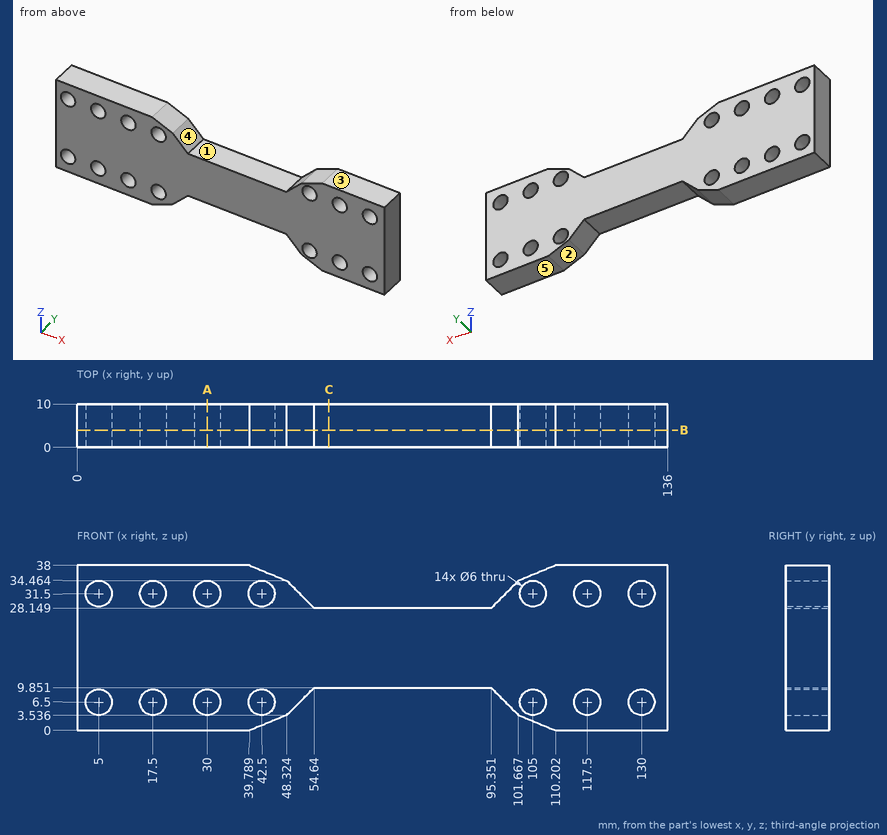
Part print with two shaded views. Sizes in mm from the minimum x, y, z corner. A direction names the side the tool comes from. Coordinates: 2 decimals unless noted, no trailing zeros. Order: outer loops, then holes, each group sorted by start corner. A loop starts at its lowest first (then second) coordinate and runs counter-clockwise, first axis right, second up. Notation, with made-up numbers: (-13.5, 39) - (22.5, 39) arc R16 cw to (22.5, 47) - close; hole circle Ø1 at (59.5, 53). An arc over 180 degrees is marked (long way). Write item = value, one per line. Start each with the question number.
1) Two-plate mould, pull along X, no slides. Class the marked faces 4 and 5: pulls with the +X half, pulls with the -X half, needs draft (parallel to the pull), parting line crosses it, or undercut.
2) Wall check: line 1 along Z through (x, y) = (44, 4) (1 decimal); line 2 along Z through (x, y) = (120, 6.75) (1 decimal); line 3 along Z through (x, y) = (57, 9.25). Give the ranges that are in metal, low to high. Write a range as from..to.
3) Flat gauge pins, fed straight in: pin 1 Ø5 at (x, z) = (30, 31.5) entering from -Y; pin 2 Ø3 at (x, y) = (72.5, 9) entering from -Z; pin 3 Ø5 at (x, y) = (71, 7.5) entering from +Z. Where does each tip first touch, or does it go through?
4) Saw through at B-B on y = 4. Count the separate pieces of the cut face and the enclosed holes in it, then the cut area to 3 significant figures.
5) 3-axis set-ups, long thin cutter, end or side, ignore diameter. For the marked faces 1, 2 and 3: which of +Z, -Z, +X, -X, +Y, -Y reach the whole face in a straight line?
6) Saw through at C-C on x = 58. Write the cut outline in (y, z), then the cut area to 3 significant figures.
7) Saw through at A-A on x = 30. Write the cut outline in (y, z), then the cut area to 3 significant figures.
From the geometry:
q1.face_4 = undercut
q1.face_5 = needs draft
q2.line_1 = 1.7..3.9, 9.1..28.9, 34.1..36.3
q2.line_2 = 0..4.8, 8.2..29.8, 33.2..38
q2.line_3 = 9.85..28.15
q3.pin_1 = through
q3.pin_2 = 9.85
q3.pin_3 = 28.15
q4.separate_pieces = 1
q4.enclosed_holes = 14
q4.area = 3,740 mm^2
q5.face_1 = +Z, +Y, -Y
q5.face_2 = -Z, +Y, -Y
q5.face_3 = +Z, +X, -X, +Y, -Y
q6.outline = (0, 9.85) - (10, 9.85) - (10, 28.15) - (0, 28.15) - close
q6.area = 183 mm^2
q7.outline = (0, 0) - (10, 0) - (10, 3.5) - (0, 3.5) - close; (0, 9.5) - (10, 9.5) - (10, 28.5) - (0, 28.5) - close; (0, 34.5) - (10, 34.5) - (10, 38) - (0, 38) - close
q7.area = 260 mm^2
